The model under review builds one solid part; all positions refer to its coordinate system, in mm. A direction names the side the tool comes from. Give positions to 0.01 mm unless a question says otherwise; leave off trailing zeros. Loops run counter-clockwise (first coordinate to the right, second up) from the corner with the lowest first, then second, coordinate; pieces in that order, holes last. Notation, with made-up numbers: (5.25, 38.25) - (52.25, 38.25) arc R28 cw to (52.25, 56.25) - close; hole circle Ø7 at (81, 22.25). An arc over 180 degrees is marked (long way). Answer as a JSON object with one key per item and string values.
from build123d import *
from OCP.BRepFilletAPI import BRepFilletAPI_MakeChamfer

# Parameters (mm, degrees)
SKETCH1_W           = 40
SKETCH1_H           = 30.000000000000004
BOSS_EXTRUDE1_DEPTH = 80
SHELL1_T            = -4
SKETCH2_W           = 10.889999999999999
SKETCH2_H           = 5
CUT_EXTRUDE1_DEPTH  = 91.97252332435328
FILLET1_R           = 1
CHAMFER1_SIZE       = 3
CHAMFER1_SIZE2      = 1.732050807568882
CUT_EXTRUDE2_DEPTH  = 95.33981132056604
SKETCH4_R           = 5.000000000000001
CUT_EXTRUDE3_DEPTH  = 5
FILLET2_R           = 1
FILLET3_R           = 10
FILLET4_R           = 3
CUT_EXTRUDE4_DEPTH  = 2


with BuildPart() as part:
    # Sketch1 → Boss-Extrude1 (new body)
    with BuildSketch(Plane.XY):
        with Locations((20, 15.000000000000002)):
            Rectangle(SKETCH1_W, SKETCH1_H)
    extrude(amount=BOSS_EXTRUDE1_DEPTH)

    # Shell1
    shell1_openings = [part.faces().sort_by_distance(p)[0] for p in [
        (20, 0, 40),
    ]]
    offset(amount=SHELL1_T, openings=shell1_openings, kind=Kind.INTERSECTION)

    # Sketch2 → Cut-Extrude1 (cut, through all)
    with BuildSketch(Plane(origin=(0, 0, 76), x_dir=(-1, 0, 0), z_dir=(0, 0, -1))):
        with Locations((-18.76162487822802, 10.397683125280034)):
            Rectangle(SKETCH2_W, SKETCH2_H)
    extrude(amount=-CUT_EXTRUDE1_DEPTH, mode=Mode.SUBTRACT)

    # Fillet1
    fillet1_edges = [part.edges().sort_by_distance(p)[0] for p in [
        (13.316624878228021, 12.897683125280034, 78),
        (13.316624878228021, 7.897683125280034, 78),
        (24.206624878228023, 7.897683125280034, 78),
        (24.206624878228023, 12.897683125280034, 78),
    ]]
    fillet(fillet1_edges, radius=FILLET1_R)

    # Chamfer1: one chamfer whose edges measure the first distance from different faces: ONE call of the kernel's chamfer builder (chamfer() names one face for all edges)
    chamfer1_edges_1 = [part.edges().sort_by_distance(p)[0] for p in [
        (13.316624878228021, 10.397683125280034, 80),
    ]]
    chamfer1_side_1 = [part.faces().sort_by_distance(p)[0] for p in [
        (13.316624878228021, 10.397683125280034, 78),
    ]]
    chamfer1_edges_2 = [part.edges().sort_by_distance(p)[0] for p in [
        (18.761624878228023, 7.897683125280034, 80),
    ]]
    chamfer1_side_2 = [part.faces().sort_by_distance(p)[0] for p in [
        (18.761624878228023, 7.897683125280035, 78),
    ]]
    chamfer1_edges_3 = [part.edges().sort_by_distance(p)[0] for p in [
        (18.761624878228023, 12.897683125280034, 80),
    ]]
    chamfer1_side_3 = [part.faces().sort_by_distance(p)[0] for p in [
        (18.761624878228023, 12.897683125280034, 78),
    ]]
    chamfer1_edges_4 = [part.edges().sort_by_distance(p)[0] for p in [
        (24.206624878228023, 10.397683125280034, 80),
    ]]
    chamfer1_side_4 = [part.faces().sort_by_distance(p)[0] for p in [
        (24.206624878228023, 10.397683125280034, 78),
    ]]
    chamfer1_edges_5 = [part.edges().sort_by_distance(p)[0] for p in [
        (13.609518097041473, 8.190576344093486, 80),
    ]]
    chamfer1_side_5 = [part.faces().sort_by_distance(p)[0] for p in [
        (13.609518097041473, 8.190576344093486, 78),
    ]]
    chamfer1_edges_6 = [part.edges().sort_by_distance(p)[0] for p in [
        (13.609518097041473, 12.604789906466582, 80),
    ]]
    chamfer1_side_6 = [part.faces().sort_by_distance(p)[0] for p in [
        (13.609518097041473, 12.604789906466582, 78),
    ]]
    chamfer1_edges_7 = [part.edges().sort_by_distance(p)[0] for p in [
        (23.91373165941457, 8.190576344093486, 80),
    ]]
    chamfer1_side_7 = [part.faces().sort_by_distance(p)[0] for p in [
        (23.91373165941457, 8.190576344093486, 78),
    ]]
    chamfer1_edges_8 = [part.edges().sort_by_distance(p)[0] for p in [
        (23.91373165941457, 12.604789906466582, 80),
    ]]
    chamfer1_side_8 = [part.faces().sort_by_distance(p)[0] for p in [
        (23.91373165941457, 12.604789906466582, 78),
    ]]
    chamfer1 = BRepFilletAPI_MakeChamfer(part.part.solid().wrapped)
    for e in chamfer1_edges_1:
        chamfer1.Add(CHAMFER1_SIZE, CHAMFER1_SIZE2, e.wrapped, chamfer1_side_1[0].wrapped)  # the first distance lies on this face
    for e in chamfer1_edges_2:
        chamfer1.Add(CHAMFER1_SIZE, CHAMFER1_SIZE2, e.wrapped, chamfer1_side_2[0].wrapped)  # the first distance lies on this face
    for e in chamfer1_edges_3:
        chamfer1.Add(CHAMFER1_SIZE, CHAMFER1_SIZE2, e.wrapped, chamfer1_side_3[0].wrapped)  # the first distance lies on this face
    for e in chamfer1_edges_4:
        chamfer1.Add(CHAMFER1_SIZE, CHAMFER1_SIZE2, e.wrapped, chamfer1_side_4[0].wrapped)  # the first distance lies on this face
    for e in chamfer1_edges_5:
        chamfer1.Add(CHAMFER1_SIZE, CHAMFER1_SIZE2, e.wrapped, chamfer1_side_5[0].wrapped)  # the first distance lies on this face
    for e in chamfer1_edges_6:
        chamfer1.Add(CHAMFER1_SIZE, CHAMFER1_SIZE2, e.wrapped, chamfer1_side_6[0].wrapped)  # the first distance lies on this face
    for e in chamfer1_edges_7:
        chamfer1.Add(CHAMFER1_SIZE, CHAMFER1_SIZE2, e.wrapped, chamfer1_side_7[0].wrapped)  # the first distance lies on this face
    for e in chamfer1_edges_8:
        chamfer1.Add(CHAMFER1_SIZE, CHAMFER1_SIZE2, e.wrapped, chamfer1_side_8[0].wrapped)  # the first distance lies on this face
    add(Compound.cast(chamfer1.Shape()), mode=Mode.REPLACE)

    # Sketch3 → Cut-Extrude2 (cut, through all)
    with BuildSketch(Plane.ZY):
        Polygon((0, 30), (22.5, 30), (22.5, 7.220000000000001), (1.47e-15, 7.220000000000001), align=None)
    extrude(amount=-CUT_EXTRUDE2_DEPTH, mode=Mode.SUBTRACT)

    # Sketch4 → Cut-Extrude3 (cut)
    with BuildSketch(Plane.XY.offset(80)):
        with Locations((20, 20.999999999999996)):
            Circle(SKETCH4_R)
    extrude(amount=-CUT_EXTRUDE3_DEPTH, mode=Mode.SUBTRACT)

    # Fillet2
    fillet2_edges = [part.edges().sort_by_distance(p)[0] for p in [
        (15, 20.999999999999996, 80),
    ]]
    fillet(fillet2_edges, radius=FILLET2_R)

    # Fillet3
    fillet3_edges = [part.edges().sort_by_distance(p)[0] for p in [
        (2, 7.220000000000001, 22.5),
        (38, 7.220000000000001, 22.5),
    ]]
    fillet(fillet3_edges, radius=FILLET3_R)

    # Fillet4
    fillet4_edges = [part.edges().sort_by_distance(p)[0] for p in [
        (40, 15, 80),
        (20, 30, 80),
        (0, 15, 80),
        (40, 3.6100000000000003, 0),
        (0, 30, 51.25),
        (40, 30, 51.25),
        (0, 3.6099999999999994, 0),
        (20, 30, 22.5),
    ]]
    fillet(fillet4_edges, radius=FILLET4_R)

    # Sketch5 → Cut-Extrude4 (cut)
    with BuildSketch(Plane.XZ):
        with BuildLine():
            Line((36.65, 78.14999999999998), (3.3499999999999988, 78.14999999999998))
            ThreePointArc((3.3499999999999988, 78.14999999999998), (2.2893398282201787, 77.7106601717798), (1.8500000000000005, 76.64999999999998))
            Line((1.8500000000000005, 76.64999999999998), (1.8500000000000096, 3.350000000000001))
            ThreePointArc((1.8500000000000096, 3.350000000000001), (2.2893398282201884, 2.2893398282201796), (3.35000000000001, 1.850000000000001))
            Line((3.35000000000001, 1.850000000000001), (36.65, 1.8500000000000028))
            ThreePointArc((36.65, 1.8500000000000028), (37.71066017177982, 2.289339828220177), (38.150000000000006, 3.350000000000003))
            Line((38.150000000000006, 3.350000000000003), (38.150000000000006, 76.64999999999998))
            ThreePointArc((38.150000000000006, 76.64999999999998), (37.71066017177982, 77.7106601717798), (36.65, 78.14999999999998))
        make_face()
        Polygon((4, 76), (4.000000000000009, 4.000000000000001), (36.00000000000001, 4.000000000000003), (36.00000000000001, 76), align=None, mode=Mode.SUBTRACT)
    extrude(amount=-CUT_EXTRUDE4_DEPTH, mode=Mode.SUBTRACT)


solid = part.part
Q1. Consider section B-B, the plane z = 9.5. State the section outline as (x, y) points, plus the area to 3 significant figures.
Results:
{"outline": "(0, 0) - (1.85, 0) - (1.85, 2) - (4, 2) - (4, 7.22) - (0, 7.22) - close; (36, 2) - (38.15, 2) - (38.15, 0) - (40, 0) - (40, 7.22) - (36, 7.22) - close", "area": "49.2 mm^2"}
Q2. The part is to be moulded in two halves that separate along Z. For faces 4 (the face through (1.85, 1, 41)), 5 (the face through (18.7, 7.02, 78.52)), 6 (the face through (2.03, 10.07, 19.49)), say which applies: +Z half, -Z half, draft (parallel to the pull), parting line (faces both ways), or undercut.
Results:
{"face 4": "undercut", "face 5": "+Z half", "face 6": "-Z half"}
Q3. Consider section A-A, the plane x = 29.5. State the section outline as (y, z) points, plus the area to 3 significant figures.
Results:
{"outline": "(0, 0) - (7.22, 0) - (7.22, 4) - (2, 4) - (2, 1.85) - (0, 1.85) - close; (0, 78.15) - (2, 78.15) - (2, 76) - (26, 76) - (26, 22.5) - (27, 22.5) arc R3 ccw to (30, 25.5) - (30, 77) arc R3 ccw to (27, 80) - (0, 80) - close", "area": "350 mm^2"}
Q4. Clearance check with flat-ended pins moving along their axes: pin 1 Ø6 at (x, z) = (33.5, 39.5) entering from -Y; pin 2 Ø5 at (x, y) = (28, 17) entering from -Z; pin 3 Ø2 at (x, z) = (32.5, 56) entering from -Y. State where each tip first meets the part, or that it passes through.
Results:
{"pin 1": "stops at y = 2", "pin 2": "stops at z = 76", "pin 3": "stops at y = 26"}
Q5. To check wall thickness, follow probe 1 along Y at (x, z) = (20, 76.8); probe 2 along X at (y, z) = (18, 51.5); probe 3 along X at (y, z) = (21, 76.7). State the ranges of each line that lie inside material, in increasing order. Write a range as [from, to].
Results:
{"probe 1": "y = [2, 7.9], [12.9, 16], [26, 30]", "probe 2": "x = [0, 4], [36, 40]", "probe 3": "x = [0, 15], [25, 40]"}
Q6. Consider section D-D, the plane y = 21. State the section outline as (x, z) points, plus the area to 3 significant figures.
Results:
{"outline": "(0, 22.5) - (4, 22.5) - (4, 76) - (15, 76) - (15, 79) arc R1 ccw to (14, 80) - (3, 80) arc R3 ccw to (0, 77) - close; (25, 76) - (36, 76) - (36, 22.5) - (40, 22.5) - (40, 77) arc R3 ccw to (37, 80) - (26, 80) arc R1 ccw to (25, 79) - close", "area": "544 mm^2"}
Q7. For faces 1 (the face through (13.003, 13.24, 78.521)), 2 (the face through (3.8, 2, 43)), 3 (the face through (0.86, 3.66, 0.9)), list the 3-axis set-ups (+Z, -Z, +X, -X, +Y, -Y) from which the entire face can be reached by the end or side of a thin tool; tool diameter is ignored.
Results:
{"face 1": "+Z", "face 2": "-Y", "face 3": "-Z, -X, +Y, -Y"}
Q8. Consider section C-C, the plane y = 3.5. State the section outline as (x, z) points, plus the area to 3 significant figures.
Results:
{"outline": "(0, 3) arc R3 ccw to (3, 0) - (37, 0) arc R3 ccw to (40, 3) - (40, 77) arc R3 ccw to (37, 80) - (3, 80) arc R3 ccw to (0, 77) - close; hole (4, 4) - (36, 4) - (36, 76) - (4, 76) - close", "area": "888 mm^2"}
